from build123d import *

# Parameters (mm, degrees)
SKETCH1_R                                        = 20
BOSS_EXTRUDE1_DEPTH                              = 6.5
CBORE_FOR_M2_PAN_HEAD_MACHINE_SCREW1_D           = 2.2
CBORE_FOR_M2_PAN_HEAD_MACHINE_SCREW1_CBORE_D     = 5
CBORE_FOR_M2_PAN_HEAD_MACHINE_SCREW1_CBORE_DEPTH = 1.6
TAP_DRILL_FOR_M4X0_7_TAP1_D                      = 3.3
SHELL1_START                                     = -6.5
SHELL1_OUTLINE_R                                 = 4.5
SHELL1_DEPTH                                     = 4.5
SHELL1_2_OUTLINE_R                               = 4.5
SHELL1_2_OUTLINE_R_2                             = 3.1
SHELL1_2_DEPTH                                   = 2.9
BOSS_EXTRUDE2_START                              = 4.5
SKETCH5_R                                        = 12
SKETCH5_R_2                                      = 1.1
BOSS_EXTRUDE2_DEPTH                              = 4.5
SKETCH6_W                                        = 1.346153846
SKETCH6_H                                        = 0.358974359
CUT_EXTRUDE1_DEPTH                               = 0.25
SKETCH7_R                                        = 0.95
BOSS_EXTRUDE3_DEPTH                              = 2.5
CUT_EXTRUDE2_DEPTH                               = 30.021543722


# Read off the part's stored shape, not the designer's step: Shell1
with BuildPart() as part:
    # Sketch1 → Boss-Extrude1 (new body)
    with BuildSketch(Plane(origin=(0, 0, 0), x_dir=(1, 0, 0), z_dir=(0, 1, 0))):
        with Locations(Location((0, 0, 0), (0, 0, 270))):
            Circle(SKETCH1_R)
    extrude(amount=-BOSS_EXTRUDE1_DEPTH)

    # CBORE for M2 Pan Head Machine Screw1 (through all)
    with Locations(Plane(origin=(3.125, 0, -5.412658774), x_dir=(0, 0, 1), z_dir=(0, 1, 0))):
        with Locations((0, 0), (5.412658774, -9.375), (10.825317548, 0)):
            CounterBoreHole(CBORE_FOR_M2_PAN_HEAD_MACHINE_SCREW1_D / 2, CBORE_FOR_M2_PAN_HEAD_MACHINE_SCREW1_CBORE_D / 2, CBORE_FOR_M2_PAN_HEAD_MACHINE_SCREW1_CBORE_DEPTH)

    # Tap Drill for M4x0.7 Tap1 (through all)
    with Locations(Plane(origin=(0, 0, 0), x_dir=(1, 0, 0), z_dir=(0, 1, 0))):
        with Locations((15, 0), (-7.5, 12.990381057), (-7.5, -12.990381057)):
            Hole(TAP_DRILL_FOR_M4X0_7_TAP1_D / 2)

    # Shell1 outline → Shell1 (cut)
    with BuildSketch(Plane(origin=(0, 0, 0), x_dir=(1, 0, 0), z_dir=(0, 1, 0)).offset(SHELL1_START)):
        with BuildLine():
            ThreePointArc((17.855916667, -2.272936425), (11.35, 0), (17.855916667, 2.272936425))
            ThreePointArc((17.855916667, 2.272936425), (9, 15.588457268), (-6.959537648, 16.600145654))
            ThreePointArc((-6.959537648, 16.600145654), (-5.675, 9.829388333), (-10.896379019, 14.327209229))
            ThreePointArc((-10.896379019, 14.327209229), (-18, 0), (-10.896379019, -14.327209229))
            ThreePointArc((-10.896379019, -14.327209229), (-5.675, -9.829388333), (-6.959537648, -16.600145654))
            ThreePointArc((-6.959537648, -16.600145654), (9, -15.588457268), (17.855916667, -2.272936425))
        make_face()
        with Locations((-6.25, 0)):
            Circle(SHELL1_OUTLINE_R, mode=Mode.SUBTRACT)
        with Locations((3.125, -5.412658774)):
            Circle(SHELL1_OUTLINE_R, mode=Mode.SUBTRACT)
        with Locations((3.125, 5.412658774)):
            Circle(SHELL1_OUTLINE_R, mode=Mode.SUBTRACT)
    extrude(amount=SHELL1_DEPTH, mode=Mode.SUBTRACT)

    # Shell1 2 outline → Shell1 2 (cut)
    # profile 1 of 3: a face of its own
    with BuildSketch(Plane(origin=(0, 0, 0), x_dir=(1, 0, 0), z_dir=(0, 1, 0)).offset(SHELL1_START)):
        with Locations((3.125, -5.412658774)):
            Circle(SHELL1_2_OUTLINE_R)
        with Locations((3.125, -5.412658774)):
            Circle(SHELL1_2_OUTLINE_R_2, mode=Mode.SUBTRACT)
    # profile 2 of 3: a face of its own
    with BuildSketch(Plane(origin=(0, 0, 0), x_dir=(1, 0, 0), z_dir=(0, 1, 0)).offset(SHELL1_START)):
        with Locations((-6.25, 0)):
            Circle(SHELL1_2_OUTLINE_R)
        with Locations((-6.25, 0)):
            Circle(SHELL1_2_OUTLINE_R_2, mode=Mode.SUBTRACT)
    # profile 3 of 3: a face of its own
    with BuildSketch(Plane(origin=(0, 0, 0), x_dir=(1, 0, 0), z_dir=(0, 1, 0)).offset(SHELL1_START)):
        with Locations((3.125, 5.412658774)):
            Circle(SHELL1_2_OUTLINE_R)
        with Locations((3.125, 5.412658774)):
            Circle(SHELL1_2_OUTLINE_R_2, mode=Mode.SUBTRACT)
    extrude(amount=SHELL1_2_DEPTH, mode=Mode.SUBTRACT)

    # Sketch5 → Boss-Extrude2 (add)
    with BuildSketch(Plane.XZ.offset(2).offset(BOSS_EXTRUDE2_START)):
        Circle(SKETCH5_R)
        with Locations(Location((3.125, -5.412658774, 0), (0, 0, 90))):
            Circle(SKETCH5_R_2, mode=Mode.SUBTRACT)
        with Locations(Location((-6.25, 0, 0), (0, 0, 90))):
            Circle(SKETCH5_R_2, mode=Mode.SUBTRACT)
        with Locations(Location((3.125, 5.412658774, 0), (0, 0, 90))):
            Circle(SKETCH5_R_2, mode=Mode.SUBTRACT)
    extrude(amount=-BOSS_EXTRUDE2_DEPTH)

    # Sketch6 → Cut-Extrude1 (cut)
    with BuildSketch(Plane(origin=(0, 0, 0), x_dir=(1, 0, 0), z_dir=(0, 1, 0))):
        Polygon((-17.309082509, 1.733907393), (-16.946602541, 1.733907393), (-16.030236355, 0.302216688), (-15.11387017, 1.733907393), (-14.751390202, 1.733907393), (-15.848645811, 0.018963483), (-14.706518407, -1.766092607), (-15.068998375, -1.766092607), (-16.030236355, -0.264289722), (-16.991474336, -1.766092607), (-17.353954304, -1.766092607), (-16.211125779, 0.018963483), align=None)
        with Locations((-13.741774817, -0.419938761)):
            Rectangle(SKETCH6_W, SKETCH6_H)
    extrude(amount=-CUT_EXTRUDE1_DEPTH, mode=Mode.SUBTRACT)

    # Sketch7 → Boss-Extrude3 (add)
    with BuildSketch(Plane.XZ.offset(6.5)):
        with Locations(Location((6.248, 0, 0), (0, 0, 90))):
            Circle(SKETCH7_R)
        with Locations(Location((-3.125, -5.410349249, 0), (0, 0, 90))):
            Circle(SKETCH7_R)
    extrude(amount=BOSS_EXTRUDE3_DEPTH)

    # Sketch9 → Cut-Extrude2 (cut, through all)
    with BuildSketch(Plane.XZ.offset(6.5)):
        with BuildLine():
            Line((-19.748437439, 0.25), (-19.748437439, -0.25))
            Line((-19.748437439, -0.25), (-19.998437439, -0.25))
            ThreePointArc((-19.998437439, -0.25), (-20, 0), (-19.998437439, 0.25))
            Line((-19.998437439, 0.25), (-19.748437439, 0.25))
        make_face()
    extrude(amount=-CUT_EXTRUDE2_DEPTH, mode=Mode.SUBTRACT)


solid = part.part
Could you check a few things on this model? Use its own coordinates, in mm. A direction names the side the tool comes from. Give positions to 0.01 mm unless a question says otherwise; leave off trailing zeros. Order: outer loops, then holes, each group sorted by start corner. A loop starts at its lowest first (then second) coordinate and runs counter-clockwise, first axis right, second up.
1. Suppose I cut it at B-B (y = -5). State how many separate pieces and enclosed holes the cut face has, plus the area to 3 significant figures.
Answers below:
separate pieces: 1
enclosed holes: 9
area: 769 mm2
2. Suppose I cut it at D-D (y = -8.5). Write out the boundary of the cut face in (x, z) (3 decimals).
Answers below:
outline: circle Ø1.9 at (-3.125, -5.41); circle Ø1.9 at (6.248, 0)
3. Thinking about a two-plate mould opening in X: for faces 1 (the cylindrical face through (5.306, -7.732, -0.124)), 2 (the cylindrical face through (9.2, -4.28, -15.47)), 3 (the flat face through (-13, -2, 0)), 4 (the flat face through (0, 0, 0)), which applies, +X half, -X half, draft (parallel to the pull), parting line (faces both ways), or undercut?
Answers below:
face 1: parting line
face 2: undercut
face 3: undercut
face 4: draft
4. For pin 1 (1.5 mm diameter, centred on x = -5.5, z = 0.5, fed in from +Y); pin 2 (11.5 mm diameter, centred on x = -14.5, z = 5, fed in from -Y); pin 3 (3 mm diameter, centred on x = 15, z = 0, fed in from -Y); pin 4 (1.5 mm diameter, centred on x = 12.5, y = -2.5, fed in from -Z), each with a flat end and sliding along its axis, tell me the tip position at first contact or that it passes through.
Answers below:
pin 1: stops at y = -1.6
pin 2: stops at y = -6.5
pin 3: passes through
pin 4: stops at z = -16.18
5. Which directions (+Z, -Z, +X, -X, +Y, -Y) give clear straight access to the entire face, cutting with the end or side of a thin tool? Please do faces 5 (the flat face through (5, -2, 12)), 6 (the flat face through (3, -1.6, -4)), 7 (the flat face through (-3, -9, -5)).
Answers below:
face 5: -Y
face 6: +Y
face 7: +Z, -Z, +X, -X, -Y
6. Suppose I cut it at C-C (z = 13.5). Write out the boundary of the cut face in (x, y).
Answers below:
outline: (-14.76, -6.5) - (-11.91, -6.5) - (-11.91, -2) - (-11.11, -2) - (-11.11, -6.5) - (-9.07, -6.5) - (-9.07, 0) - (-14.76, 0) - close; (-5.93, -6.5) - (-3.89, -6.5) - (-3.89, -2) - (11.91, -2) - (11.91, -6.5) - (14.76, -6.5) - (14.76, 0) - (-5.93, 0) - close
7. I need wall thicknesses on L1, parallel to Z at x = -5, y = -5; L2, parallel to Z at x = 16, y = -3; L3, parallel to Z at x = 6, y = -6. Which ranges of each line are inside material? Lowest first, please.
Answers below:
L1: z = -19.36 to -17.29, -15.65 to 15.65, 17.29 to 19.36
L2: z = -12 to -8.25, -3.51 to -1.31, 1.31 to 3.51, 8.25 to 12
L3: z = -19.08 to -16.97, -10.39 to 10.39, 16.97 to 19.08
8. Suppose I cut it at A-A (x = 15). Write out the boundary of the cut face in (y, z), plus the area to 3 significant figures.
Answers below:
outline: (-6.5, -13.23) - (0, -13.23) - (0, -1.65) - (-6.5, -1.65) - (-6.5, -3.65) - (-2, -3.65) - (-2, -9.95) - (-6.5, -9.95) - close; (-6.5, 1.65) - (0, 1.65) - (0, 13.23) - (-6.5, 13.23) - (-6.5, 9.95) - (-2, 9.95) - (-2, 3.65) - (-6.5, 3.65) - close
area: 93.8 mm2
